from build123d import *

# Parameters (mm, degrees)
SKETCH1_R                                         = 15
SKETCH1_R_2                                       = 5.5
BODY_DEPTH                                        = 3.175
CSK_FOR_6_FLAT_HEAD_MACHINE_SCREW_100_D           = 3.7973
CSK_FOR_6_FLAT_HEAD_MACHINE_SCREW_100_CSINK_D     = 7.0866
CSK_FOR_6_FLAT_HEAD_MACHINE_SCREW_100_CSINK_ANGLE = 100


with BuildPart() as part:
    # Sketch1 → Body (new body)
    with BuildSketch(Plane.XY):
        Circle(SKETCH1_R)
        Circle(SKETCH1_R_2, mode=Mode.SUBTRACT)
    extrude(amount=BODY_DEPTH)

    # CSK for #6 Flat Head Machine Screw (100)1 (through all)
    with Locations(Plane(origin=(0, 10, 3.175), x_dir=(1, 0, 0), z_dir=(0, 0, 1))):
        with Locations((0, 0), (-8.660254038, -15), (8.660254038, -15)):
            CounterSinkHole(CSK_FOR_6_FLAT_HEAD_MACHINE_SCREW_100_D / 2, CSK_FOR_6_FLAT_HEAD_MACHINE_SCREW_100_CSINK_D / 2, counter_sink_angle=CSK_FOR_6_FLAT_HEAD_MACHINE_SCREW_100_CSINK_ANGLE)


solid = part.part
For this review, take the finished solid that the model builds, in its own axes (mm). Round coordinates to 2 decimals unless told otherwise and drop trailing zeros. Write each loop counter-clockwise with the first axis right and the second up, starting at its lowest first coordinate (ties: lowest second). Pieces come first, ordered by that corner, then holes. Notation, with made-up numbers: (22, -28.75) -> (33, -28.75) arc R28 ccw to (33, 1.25) -> close; hole circle Ø3 at (12, 72.25). An arc over 180 degrees is marked (long way). Use CSV: the item, a comma, the result in double quotes.
(1) Consider section D-D, the plane y = 10. Give the boundary of the cut face in (x, z) (3 decimals).
Computed values:
outline,"(-11.18, 0) -> (-1.899, 0) -> (-1.899, 1.795) -> (-3.543, 3.175) -> (-11.18, 3.175) -> close; (1.899, 0) -> (11.18, 0) -> (11.18, 3.175) -> (3.543, 3.175) -> (1.899, 1.795) -> close"
(2) Draft analysis for pull direction X (two halves, no side actions). For faces 1 (the face through (-14.985, 0.66, 1.565)), 2 (the face through (6.85, -4.43, 0.88)), 3 (the face through (0.247, 11.882, 0.885)), 4 (the face through (6, 0, 3.175)), state which applies: +X half, -X half, draft (parallel to the pull), parting line (faces both ways), or undercut.
Computed values:
face 1,"parting line"
face 2,"undercut"
face 3,"undercut"
face 4,"draft"
(3) Consider section B-B, the plane z = 1.25. Give the boundary of the cut face in (x, y), plus the area to 3 significant figures.
Computed values:
outline,"circle Ø30 at (0, 0); hole circle Ø3.8 at (-8.66, -5); hole circle Ø11 at (0, 0); hole circle Ø3.8 at (0, 10); hole circle Ø3.8 at (8.66, -5)"
area,"578 mm²"
(4) To check wall thickness, follow L1, parallel to Y at x = 0, z = 1.2; L2, parallel to Y at x = 1.5, z = 0.75; L3, parallel to X at y = -5.75, z = 0.8. State the ranges of each line that lie inside material, in increasing order. Write a range as [from, to].
Computed values:
L1,"[-15, -5.5], [5.5, 8.1], [11.9, 15]"
L2,"[-14.92, -5.29], [5.29, 8.84], [11.16, 14.92]"
L3,"[-13.85, -10.4], [-6.92, 6.92], [10.4, 13.85]"
(5) Consider section C-C, the plane y = -5. Give the boundary of the cut face in (x, z) (3 decimals), plus the area to 3 significant figures.
Computed values:
outline,"(-14.142, 0) -> (-10.559, 0) -> (-10.559, 1.795) -> (-12.204, 3.175) -> (-14.142, 3.175) -> close; (-6.762, 0) -> (-2.291, 0) -> (-2.291, 3.175) -> (-5.117, 3.175) -> (-6.762, 1.795) -> close; (2.291, 0) -> (6.762, 0) -> (6.762, 1.795) -> (5.117, 3.175) -> (2.291, 3.175) -> close; (10.559, 0) -> (14.142, 0) -> (14.142, 3.175) -> (12.204, 3.175) -> (10.559, 1.795) -> close"
area,"46.6 mm²"
(6) Clearance check with flat-ended pins moving along their axes: P1, Ø4.5, axis at x = -8.66, y = -5, coming from the +Z side; P2, Ø1.5, axis at x = -10.5, z = 2.5, coming from the -Y side. State where each tip first meets the part, or that it passes through.
Computed values:
P1,"z = 2.09"
P2,"y = -11.4"
(7) Consider section A-A, the plane y = 2.5. Give the boundary of the cut face in (x, z) (3 decimals), plus the area to 3 significant figures.
Computed values:
outline,"(-14.79, 0) -> (-4.899, 0) -> (-4.899, 3.175) -> (-14.79, 3.175) -> close; (4.899, 0) -> (14.79, 0) -> (14.79, 3.175) -> (4.899, 3.175) -> close"
area,"62.8 mm²"
